Geometry check sheet. Reference: the model listing, model coordinates, mm. Round coordinates to 2 decimals unless told otherwise and drop trailing zeros. Order: outer loops, then holes, each group sorted by start corner. A loop starts at its lowest first (then second) coordinate and runs counter-clockwise, first axis right, second up.
```python
from build123d import *

# Parameters (mm, degrees)
STRUCTURE_SYSTEM1_OUTLINE_R   = 13.45
STRUCTURE_SYSTEM1_OUTLINE_R_2 = 10.25
STRUCTURE_SYSTEM1_DEPTH       = 1000
CUT_EXTRUDE1_DEPTH            = 1001.18088614
CUT_EXTRUDE1_DEPTH_BACK       = 1001.18088614
SKETCH12_R                    = 7.5


# Read off the part's stored shape, not the designer's step: Structure System1
with BuildPart() as part:
    # Structure System1 outline → Structure System1 (new body)
    with BuildSketch(Plane(origin=(0, 0, 0), x_dir=(1, 0, 0), z_dir=(0, 1, 0))):
        Circle(STRUCTURE_SYSTEM1_OUTLINE_R)
        Circle(STRUCTURE_SYSTEM1_OUTLINE_R_2, mode=Mode.SUBTRACT)
    extrude(amount=STRUCTURE_SYSTEM1_DEPTH)

    # Sketch12 → Cut-Extrude1 (cut, two sides: drawn at the far end of the back side and taken through both)
    with BuildSketch(Plane(origin=(0, 0, 0), x_dir=(0, 0, -1), z_dir=(1, 0, 0)).offset(-CUT_EXTRUDE1_DEPTH_BACK)):
        with Locations((0, 639.041378949)):
            Circle(SKETCH12_R)
    extrude(amount=CUT_EXTRUDE1_DEPTH + CUT_EXTRUDE1_DEPTH_BACK, mode=Mode.SUBTRACT)


solid = part.part
```
(1) Sectioned sample at C-C, the plane y = 913. Record the cut outline in (x, z), and give its area (3 significant figures).
Returned:
outline: circle Ø26.9 at (0, 0); hole circle Ø20.5 at (0, 0)
area: 238 mm2
(2) Sectioned sample at A-A, the plane z = 0. Record the cut outline in (x, y).
Returned:
outline: (-13.45, 0) - (-10.25, 0) - (-10.25, 631.54) - (-13.45, 631.54) - close; (-13.45, 646.54) - (-10.25, 646.54) - (-10.25, 1000) - (-13.45, 1000) - close; (10.25, 0) - (13.45, 0) - (13.45, 631.54) - (10.25, 631.54) - close; (10.25, 646.54) - (13.45, 646.54) - (13.45, 1000) - (10.25, 1000) - close
(3) Sectioned sample at B-B, the plane x = -2.75. Record the cut outline in (y, z), and give its area (3 significant figures).
Returned:
outline: (0, -13.17) - (1000, -13.17) - (1000, -9.87) - (0, -9.87) - close; (0, 9.87) - (1000, 9.87) - (1000, 13.17) - (0, 13.17) - close
area: 6,580 mm2
(4) Material ranges on line 1 (X direction, y = 212, z = 0); line 2 (Z direction, x = -5.75, y = 86.5), recorded low to high.
Returned:
line 1: x = -13.45 to -10.25, 10.25 to 13.45
line 2: z = -12.16 to -8.49, 8.49 to 12.16
(5) Depth check by flat-ended pin: P1, Ø9, axis at y = 639.04, z = 0, coming from the +X side; P2, Ø8, axis at x = 4.5, y = 142.5, coming from the +Z side; P3, Ø3, axis at x = 6.5, y = 349.5, coming from the -Z side; P4, Ø3, axis at y = 861, z = 2.5, coming from the -X side. Enter the tip coordinate at first touch or a pass-through.
Returned:
P1: passes through
P2: stops at z = 13.44
P3: stops at z = -12.49
P4: stops at x = -13.41
(6) Draft check along X on faces 1 (the cylindrical face through (12.83, 493, -4.04)), 2 (the flat face through (-3, 0, 10)), 3 (the cylindrical face through (-2.222, 493, 10.006)). Enter one of: released by +X, released by -X, zero draft, split by the parting line, or undercut.
Returned:
face 1: split by the parting line
face 2: zero draft
face 3: undercut
